Geometry: see drawing. Coordinates: mm, zero at the bounding-box minimum. A direction names the side the tool comes from. Give positions to 0.01 mm unless a question says otherwise; leave off trailing zeros. Write each loop counter-clockwise with the first axis right and the second up, starting at its lowest first coordinate (ties: lowest second). Pieces come first, ordered by that corner, then holes. Notation, with made-up numbers: (-4.5, 69) -> (37.5, 69) arc R24 ccw to (37.5, 91) -> close; hole circle Ø8 at (39, -32.75). An arc over 180 degrees is marked (long way). Use CSV: the item, a comma, the result in double quotes. Start each with the question number.
1) Section D-D (x = 22.5). Output: boundary loops of the cut face in (y, z), plus the area to 3 significant figures.
2) Material intervals for line 1 (Y direction, x = 16, z = 0.5); line 2 (Y direction, x = 8.5, z = 4); line 3 (X direction, y = 26, z = 0.75), sorted ascending. Write a range as [from, to].
3) Section A-A (x = 16). Output: boundary loops of the cut face in (y, z), plus the area to 3 significant figures.
4) Contact query for flat-ended pins moving along their axis: P1, Ø20, axis at x = 23, y = 28, coming from the +Z side; P2, Ø5, axis at x = 25, z = 5, coming from the +Y side; P3, Ø3, axis at x = 15.5, y = 11, coming from the -Z side; P4, Ø1, axis at x = 27.5, z = 9.5, coming from the -Y side. Output: stop coordinate, or through.
5) Section C-C (z = 7.5). Output: boundary loops of the cut face in (x, y).
6) Set-up query: the marked faces 1, 2 and 3. Return all of +Z, -Z, +X, -X, +Y, -Y with unobstructed straight access to the full face (end or side cutting, diameter ignored); none if empty.
7) Section B-B (y = 41.5). Output: boundary loops of the cut face in (x, z), plus the area to 3 significant figures.
8) Draft query along Y for the marked faces 4, 5 and 6. Return one class per face: pulls with the +Y half, pulls with the -Y half, needs draft (parallel to the pull), parting line crosses it, or undercut.
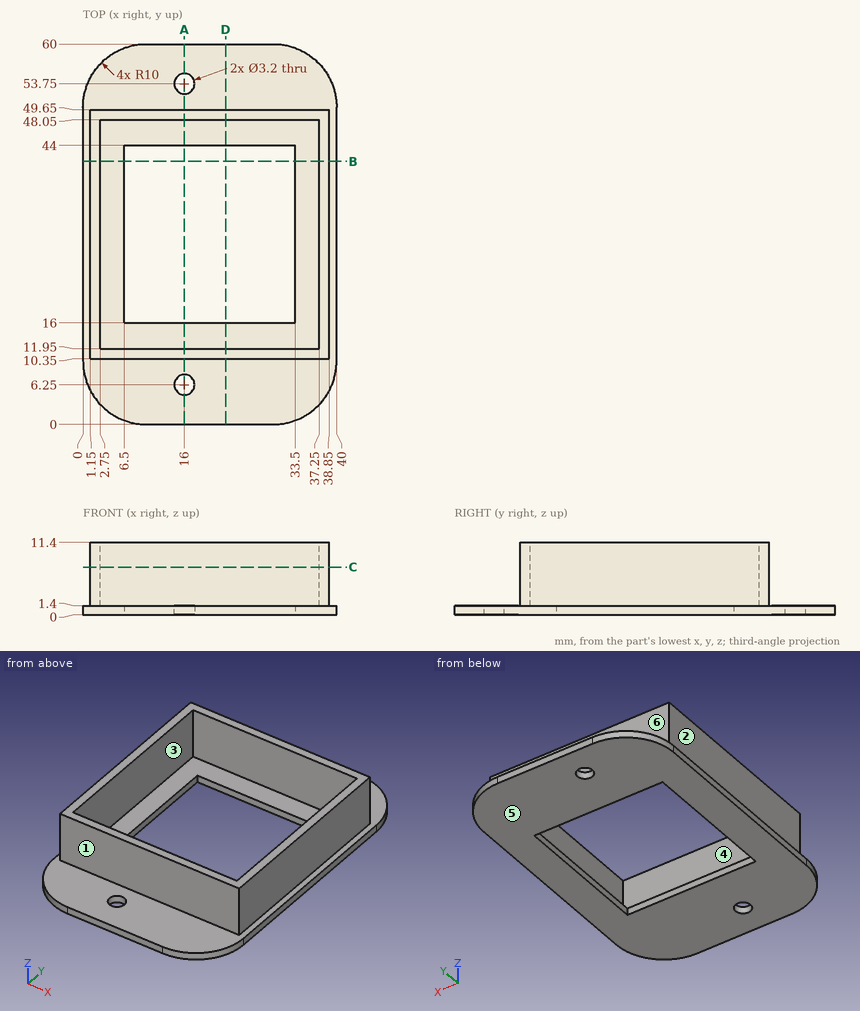
Answers follow:
1,outline,"(0, 0) -> (16, 0) -> (16, 1.4) -> (11.95, 1.4) -> (11.95, 11.4) -> (10.35, 11.4) -> (10.35, 1.4) -> (0, 1.4) -> close; (44, 0) -> (60, 0) -> (60, 1.4) -> (49.65, 1.4) -> (49.65, 11.4) -> (48.05, 11.4) -> (48.05, 1.4) -> (44, 1.4) -> close"
1,area,"76.8 mm^2"
2,line 1,"y = [0, 4.65], [7.85, 16], [44, 52.15], [55.35, 60]"
2,line 2,"y = [10.35, 11.95], [48.05, 49.65]"
2,line 3,"x = [0, 6.5], [33.5, 40]"
3,outline,"(0, 0) -> (4.65, 0) -> (4.65, 1.4) -> (0, 1.4) -> close; (7.85, 0) -> (16, 0) -> (16, 1.4) -> (11.95, 1.4) -> (11.95, 11.4) -> (10.35, 11.4) -> (10.35, 1.4) -> (7.85, 1.4) -> close; (44, 0) -> (52.15, 0) -> (52.15, 1.4) -> (49.65, 1.4) -> (49.65, 11.4) -> (48.05, 11.4) -> (48.05, 1.4) -> (44, 1.4) -> close; (55.35, 0) -> (60, 0) -> (60, 1.4) -> (55.35, 1.4) -> close"
3,area,"67.8 mm^2"
4,P1,"passes through"
4,P2,"stops at y = 49.65"
4,P3,"stops at z = 0"
4,P4,"stops at y = 10.35"
5,outline,"(1.15, 10.35) -> (38.85, 10.35) -> (38.85, 49.65) -> (1.15, 49.65) -> close; hole (2.75, 11.95) -> (37.25, 11.95) -> (37.25, 48.05) -> (2.75, 48.05) -> close"
6,face 1,"+Z, +X, -X, -Y"
6,face 2,"+Z, -X, +Y, -Y"
6,face 3,"+Z"
7,outline,"(0, 0) -> (6.5, 0) -> (6.5, 1.4) -> (2.75, 1.4) -> (2.75, 11.4) -> (1.15, 11.4) -> (1.15, 1.4) -> (0, 1.4) -> close; (33.5, 0) -> (40, 0) -> (40, 1.4) -> (38.85, 1.4) -> (38.85, 11.4) -> (37.25, 11.4) -> (37.25, 1.4) -> (33.5, 1.4) -> close"
7,area,"50.2 mm^2"
8,face 4,"undercut"
8,face 5,"needs draft"
8,face 6,"pulls with the +Y half"
